from build123d import *

# Parameters (mm, degrees)
F0_W     = 70
F0_H     = 100
F1_DEPTH = 3
F3_DEPTH = 28
F4_W     = 2
F4_H     = 78
F5_DEPTH = 30.6
F7_DEPTH = 25
F8_W     = 14.5
F8_H     = 20
F9_DEPTH = 1


with BuildPart() as f1:
    # F0 (on Top) → F1 (new body)
    with BuildSketch(Plane.XY):
        with Locations((-25.664028, 6.657216)):
            Rectangle(F0_W, F0_H)
    extrude(amount=F1_DEPTH)

    # F2 (on face) → F3 (join)
    with BuildSketch(Plane.XY.offset(3)):
        Polygon((-60.664028, -21.342784), (-60.664028, -43.342784), (9.335972, -43.342784), (9.335972, -21.342784), (7.335972, -21.342784), (7.335972, -41.342784), (-58.664028, -41.342784), (-58.664028, -21.342784), align=None)
    extrude(amount=F3_DEPTH)

    # F4 (on face) → F5 (cut)
    with BuildSketch(Plane.XY.offset(3)):
        with Locations((8.335972, 17.657216)):
            Rectangle(F4_W, F4_H)
        with Locations((-59.664028, 17.657216)):
            Rectangle(F4_W, F4_H)
    extrude(amount=-F5_DEPTH, mode=Mode.SUBTRACT)

    # F6 (on face) → F7 (cut)
    with BuildSketch(Plane(origin=(0, 0, 0), x_dir=(1, 0, 0), z_dir=(0, 0, -1))):
        Polygon((-4.164028, 21.016594), (-47.164028, 21.016594), (-47.164028, -41.657216), (-32.914028, -41.657216), (-32.914028, -21.657216), (-25.664028, -21.657216), (-18.414028, -21.657216), (-18.414028, -41.657216), (-4.164028, -41.657216), align=None)
    extrude(amount=-F7_DEPTH, mode=Mode.SUBTRACT)

    # F8 (on face) → F9 (cut)
    with BuildSketch(Plane.XY.offset(3)):
        with Locations((-25.664028, 31.657216)):
            Rectangle(F8_W, F8_H)
    extrude(amount=-F9_DEPTH, mode=Mode.SUBTRACT)


solid = f1.part
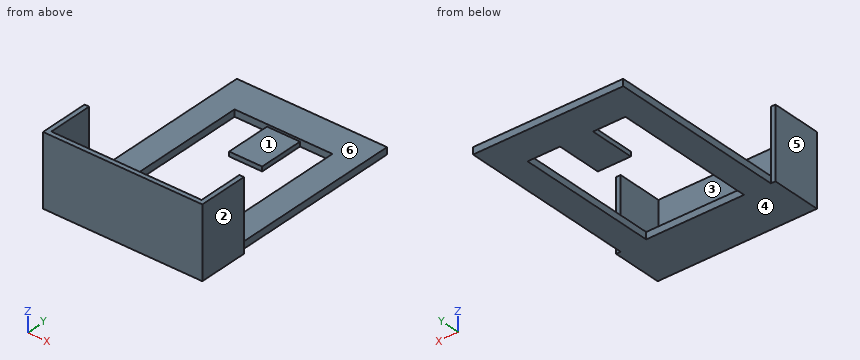
Design review of the part built by this model. Coordinates are the model's own, in mm. Face numbers are marked on the shaded views. A direction names the side the tool comes from. Round coordinates to 2 decimals unless told otherwise and drop trailing zeros. Loops run counter-clockwise (first coordinate to the right, second up) from the corner with the lowest first, then second, coordinate; pieces in that order, holes last. Notation, with made-up numbers: M 61.25,28.5 L 90.25,28.5 A26 cw 90.25,62.5 Z; hole C -9,3 d9. An arc over 180 degrees is marked long. Answer as a JSON object with one key per item and string values.
Item 1: Machinability: for the marked faces 1, 2 and 3, which of the approach directions +Z, -Z, +X, -X, +Y, -Y give a long, thin tool a straight path to every point of the face, cutting with its end or side? Answer none if there is none.
Answer sheet:
{"face 1": "+Z", "face 2": "+Z, -Z, +X, +Y, -Y", "face 3": "+Z, +Y"}
Item 2: We need section D-D on y = 15.5. Give the boundary of the cut face in (x, z), and give its area (3 significant figures).
Answer sheet:
{"outline": "M -58.66,0 L -47.16,0 L -47.16,3 L -58.66,3 Z; M -4.16,0 L 7.34,0 L 7.34,3 L -4.16,3 Z", "area": "69.0 mm^2"}
Item 3: We need section B-B on y = 33. Give the boundary of the cut face in (x, z).
Answer sheet:
{"outline": "M -58.66,0 L -47.16,0 L -47.16,3 L -58.66,3 Z; M -32.91,0 L -18.41,0 L -18.41,2 L -32.91,2 Z; M -4.16,0 L 7.34,0 L 7.34,3 L -4.16,3 Z"}
Item 4: Clearance check with flat-ended pins moving along their axes: P1, Ø1, axis at y = 36.5, z = 1.5, coming from the +X side; P2, Ø1.6, axis at x = -59.5, z = 11.5, coming from the +Y side; P3, Ø4.5, axis at x = -23, y = 31.5, coming from the +Z side. State where each tip first meets the part, or that it passes through.
Answer sheet:
{"P1": "stops at x = 7.34", "P2": "stops at y = -21.34", "P3": "stops at z = 2"}
Item 5: We need section A-A on x = -23.5. Give the boundary of the cut face in (y, z).
Answer sheet:
{"outline": "M -43.34,0 L -21.02,0 L -21.02,3 L -41.34,3 L -41.34,31 L -43.34,31 Z; M 21.66,0 L 56.66,0 L 56.66,3 L 41.66,3 L 41.66,2 L 21.66,2 Z"}
Item 6: We need section C-C on z = 13.5. Give the boundary of the cut face in (x, y), and give its area (3 significant figures).
Answer sheet:
{"outline": "M -60.66,-43.34 L 9.34,-43.34 L 9.34,-21.34 L 7.34,-21.34 L 7.34,-41.34 L -58.66,-41.34 L -58.66,-21.34 L -60.66,-21.34 Z", "area": "220 mm^2"}
Item 7: The part is to be moulded in two halves that separate along X. For the marked faces 4, 5 and 6, say which applies: pulls with the +X half, pulls with the -X half, needs draft (parallel to the pull), parting line crosses it, or undercut.
Answer sheet:
{"face 4": "needs draft", "face 5": "pulls with the -X half", "face 6": "undercut"}
Item 8: Wall thickness on L1, parallel to X at y = 35, z = 2.5; L2, parallel to Y at x = -5, z = 9; L3, parallel to X at y = -32, z = 6.5: over which ranges is each line inside the solid? List them lowest first. Write a range as from..to.
Answer sheet:
{"L1": "x = -58.66..-47.16, -4.16..7.34", "L2": "y = -43.34..-41.34", "L3": "x = -60.66..-58.66, 7.34..9.34"}
